The listing builds one solid part. Answer for the finished solid, in the listing's coordinates (mm). A direction names the side the tool comes from. Coordinates: 2 decimals unless noted, no trailing zeros. Order: outer loops, then holes, each group sorted by start corner. A loop starts at its lowest first (then second) coordinate and runs counter-clockwise, first axis right, second up. Notation, with made-up numbers: (-28, 51) -> (-22, 51) arc R24 ccw to (-22, 87) -> close; hole circle Ø7 at (-24, 52). An arc over 180 degrees is marked (long way). Write each question's results on one line, items separated by ' | '. Start each with the question number.
(1) The part is cut by section A-A, the plane z = 22.5. Give the vertices of the cut face in (x, y).
(2) Determine the mould class of faces 6 (the face through (11.64, 11.6, 1.48)), 7 (the face through (-44, 4, 26)), 8 (the face through (-68, 14, 23)) for opening direction X: +X half, -X half, draft (parallel to the pull), parting line (faces both ways), or undercut.
(3) The part is cut by section B-B, the plane z = 8.5. Count the separate pieces of the cut face and the enclosed holes in it, then the cut area to 3 significant figures.
(4) Given pin 1 (2.5 mm diameter, centred on x = 17.5, z = 1.5, fed in from -Y); pin 2 (1 mm diameter, centred on y = 27.5, z = 6.5, fed in from +X); pin 3 (5 mm diameter, centred on y = 1.5, z = 19.5, fed in from -X), each flat-ended and moving along its own axis, determine where each tip first touches the part or whether it passes through.
(5) Straight lines are drawn through the part: L1, parallel to Z at x = 8, y = 26; L2, parallel to Z at x = -18, y = 26; L3, parallel to Y at x = 0, z = 8.75. For each, find the intervals that lie inside material, in ascending order.
(6) A tool of negligible diameter and unlimited length cuts with its end or side. For faces 1 (the face through (-9, -9.07, 4.01)), 2 (the face through (-29.97, 1.32, 7.46)), 3 (the face through (-55, 15, 15)), 4 (the face through (-13.36, 5.9, 1.48)), 5 (the face through (-48, -14, 2)), from which of +Z, -Z, +X, -X, +Y, -Y can it reach the whole face along a straight path? Write none if from no direction.
```python
from build123d import *

# Parameters (mm, degrees)
BOSS_EXTRU_1_DEPTH      = 5
ESQUISSE6_R             = 34.8
ESQUISSE6_R_2           = 30
BOSS_EXTRU_6_DEPTH      = 5
BOSS_EXTRU_9_DEPTH      = 21
CONG_1_R                = 20
CONG_2_R                = 5
ESQUISSE11_W            = 20.2
ESQUISSE11_H            = 20.2
ENL_V_MAT_EXTRU_2_DEPTH = 25
ESQUISSE12_R            = 2.6
ENL_V_MAT_EXTRU_3_DEPTH = 81.987161213
ENL_V_START             = -5
ESQUISSE13_R            = 4.5
ENL_V_MAT_EXTRU_4_DEPTH = 76.987161213
ENL_V_MAT_EXTRU_5_DEPTH = 2
ENL_V_MAT_EXTRU_7_DEPTH = 3
ESQUISSE19_R            = 1.65
ENL_V_MAT_EXTRU_8_DEPTH = 83.674725752
ENL_V_MAT_EXTRU_9_DEPTH = 1


with BuildPart() as part:
    # Esquisse1 → Boss.-Extru.1 (new body)
    with BuildSketch(Plane.XY):
        with BuildLine():
            Line((-45.620718977, 15), (-70, 15))
            Line((-70, 15), (-70, -15))
            Line((-70, -15), (-45.620718977, -15))
            ThreePointArc((-45.620718977, -15), (-36.774201608, -17.062911874), (-29.752642811, -22.826086957))
            ThreePointArc((-29.752642811, -22.826086957), (37.5, 0), (-29.752642811, 22.826086957))
            ThreePointArc((-29.752642811, 22.826086957), (-36.774201608, 17.062911874), (-45.620718977, 15))
        make_face()
    extrude(amount=BOSS_EXTRU_1_DEPTH)

    # Esquisse6 → Boss.-Extru.6 (add)
    with BuildSketch(Plane.XY.offset(5)):
        Circle(ESQUISSE6_R)
        Circle(ESQUISSE6_R_2, mode=Mode.SUBTRACT)
    extrude(amount=BOSS_EXTRU_6_DEPTH)

    # Esquisse8 → Boss.-Extru.9 (add)
    with BuildSketch(Plane.XY.offset(5)):
        with BuildLine():
            Line((-70, -15), (-70, 15))
            Line((-70, 15), (-43.874821937, 15))
            ThreePointArc((-43.874821937, 15), (-39.966142137, 13.118047822), (-38.999841722, 8.888888889))
            ThreePointArc((-38.999841722, 8.888888889), (-40, 0), (-38.999841722, -8.888888889))
            ThreePointArc((-38.999841722, -8.888888889), (-39.966142137, -13.118047822), (-43.874821937, -15))
            Line((-43.874821937, -15), (-70, -15))
        make_face()
    extrude(amount=BOSS_EXTRU_9_DEPTH)

    # Congé1
    cong_1_edges = [part.edges().sort_by_distance(p)[0] for p in [
        (-70, 0, 0),
    ]]
    fillet(cong_1_edges, radius=CONG_1_R)

    # Congé2
    cong_2_edges = [part.edges().sort_by_distance(p)[0] for p in [
        (-47.810359489, -15, 0),
        (-36.774201608, -17.062911874, 0),
        (37.5, 0, 0),
        (-36.774201608, 17.062911874, 0),
        (-47.810359489, 15, 0),
        (-64.142135624, 15, 5.857864376),
        (-64.142135624, -15, 5.857864376),
        (-70, -15, 23),
        (-70, 15, 23),
    ]]
    fillet(cong_2_edges, radius=CONG_2_R - 0.0001)  # a hair under: the kernel refuses the full size

    # Esquisse11 → Enlèv. mat.-Extru.2 (cut)
    with BuildSketch(Plane.ZY.offset(70)):
        with Locations((26, 0)):
            Rectangle(ESQUISSE11_W, ESQUISSE11_H)
    extrude(amount=-ENL_V_MAT_EXTRU_2_DEPTH, mode=Mode.SUBTRACT)

    # Esquisse12 → Enlèv. mat.-Extru.3 (cut, through all)
    with BuildSketch(Plane.XY.offset(15.9)):
        with Locations((-49.575239462, 0)):
            Circle(ESQUISSE12_R)
    extrude(amount=-ENL_V_MAT_EXTRU_3_DEPTH, mode=Mode.SUBTRACT)

    # Esquisse13 → Enlèv. mat.-Extru.4 (cut, through all)
    with BuildSketch(Plane.XY.offset(15.9).offset(ENL_V_START)):
        with Locations((-49.575239462, 0)):
            Circle(ESQUISSE13_R)
    extrude(amount=-ENL_V_MAT_EXTRU_4_DEPTH, mode=Mode.SUBTRACT)

    # Esquisse14 → Enlèv. mat.-Extru.5 (cut)
    with BuildSketch(Plane.XY.offset(5)):
        with BuildLine():
            Line((-5.5, 10.5), (5.5, 10.5))
            ThreePointArc((5.5, 10.5), (9.035533906, 9.035533906), (10.5, 5.5))
            Line((10.5, 5.5), (10.5, -5.5))
            ThreePointArc((10.5, -5.5), (9.035533906, -9.035533906), (5.5, -10.5))
            Line((5.5, -10.5), (-5.5, -10.5))
            ThreePointArc((-5.5, -10.5), (-9.035533906, -9.035533906), (-10.5, -5.5))
            Line((-10.5, -5.5), (-10.5, 5.5))
            ThreePointArc((-10.5, 5.5), (-9.035533906, 9.035533906), (-5.5, 10.5))
        make_face()
    extrude(amount=-ENL_V_MAT_EXTRU_5_DEPTH, mode=Mode.SUBTRACT)

    # Esquisse17 → Enlèv. mat.-Extru.7 (cut)
    with BuildSketch(Plane(origin=(0, 0, 0), x_dir=(-1, 0, 0), z_dir=(0, 0, -1))):
        with BuildLine():
            Line((15.5, 5), (19.5, 5))
            ThreePointArc((19.5, 5), (21.621320344, 4.121320344), (22.5, 2))
            Line((22.5, 2), (22.5, -2))
            ThreePointArc((22.5, -2), (21.621320344, -4.121320344), (19.5, -5))
            Line((19.5, -5), (15.5, -5))
            ThreePointArc((15.5, -5), (13.378679656, -5.878679656), (12.5, -8))
            Line((12.5, -8), (12.5, -9.5))
            ThreePointArc((12.5, -9.5), (11.621320344, -11.621320344), (9.5, -12.5))
            Line((9.5, -12.5), (-9.5, -12.5))
            ThreePointArc((-9.5, -12.5), (-11.621320344, -11.621320344), (-12.5, -9.5))
            Line((-12.5, -9.5), (-12.5, -8))
            ThreePointArc((-12.5, -8), (-13.378679656, -5.878679656), (-15.5, -5))
            Line((-15.5, -5), (-19.5, -5))
            ThreePointArc((-19.5, -5), (-21.621320344, -4.121320344), (-22.5, -2))
            Line((-22.5, -2), (-22.5, 2))
            ThreePointArc((-22.5, 2), (-21.621320344, 4.121320344), (-19.5, 5))
            Line((-19.5, 5), (-15.5, 5))
            ThreePointArc((-15.5, 5), (-13.378679656, 5.878679656), (-12.5, 8))
            Line((-12.5, 8), (-12.5, 9.5))
            ThreePointArc((-12.5, 9.5), (-11.621320344, 11.621320344), (-9.5, 12.5))
            Line((-9.5, 12.5), (9.5, 12.5))
            ThreePointArc((9.5, 12.5), (11.621320344, 11.621320344), (12.5, 9.5))
            Line((12.5, 9.5), (12.5, 8))
            ThreePointArc((12.5, 8), (13.378679656, 5.878679656), (15.5, 5))
        make_face()
    extrude(amount=-ENL_V_MAT_EXTRU_7_DEPTH, mode=Mode.SUBTRACT)

    # Esquisse19 → Enlèv. mat.-Extru.8 (cut, through all)
    with BuildSketch(Plane(origin=(0, 0, 3), x_dir=(-1, 0, 0), z_dir=(0, 0, -1))):
        with Locations((17.5, 0)):
            Circle(ESQUISSE19_R)
        with Locations(Location((-17.5, 0, 0), (0, 0, 180))):
            Circle(ESQUISSE19_R)
    extrude(amount=-ENL_V_MAT_EXTRU_8_DEPTH, mode=Mode.SUBTRACT)

    # Esquisse20 → Enlèv. mat.-Extru.9 (cut)
    with BuildSketch(Plane.XY.offset(5)):
        Polygon((-17.5, -3.464101615), (-14.5, -1.732050808), (-14.5, 1.732050808), (-17.5, 3.464101615), (-20.5, 1.732050808), (-20.5, -1.732050808), align=None)
        Polygon((20.5, -1.732050808), (17.5, -3.464101615), (14.5, -1.732050808), (14.5, 1.732050808), (17.5, 3.464101615), (20.5, 1.732050808), align=None)
    extrude(amount=-ENL_V_MAT_EXTRU_9_DEPTH, mode=Mode.SUBTRACT)


solid = part.part
```
Established:
1) outline: (-70, -10.1) arc R5 ccw to (-65, -15) -> (-43.87, -15) arc R5 ccw to (-39, -8.89) arc R40 cw to (-39, 8.89) arc R5 ccw to (-43.87, 15) -> (-65, 15) arc R5 ccw to (-70, 10.1) -> (-45, 10.1) -> (-45, -10.1) -> close
2) face 6: undercut | face 7: draft | face 8: -X half
3) separate pieces: 2 | enclosed holes: 2 | area: 1,700 mm^2
4) pin 1: stops at y = -32.8 | pin 2: stops at x = 21.96 | pin 3: stops at x = -45
5) L1: z = 0 to 5 | L2: z = 0 to 10 | L3: y = -34.8 to -30, 30 to 34.8
6) face 1: +Z, -Z | face 2: +Z | face 3: +Z, -Z, -X, +Y | face 4: -Z | face 5: -Z, -X, -Y
